Build history of the part. All positions in model axes, mm. A direction names the side the tool comes from. Round coordinates to 2 decimals unless told otherwise and drop trailing zeros. Write each loop counter-clockwise with the first axis right and the second up, starting at its lowest first coordinate (ties: lowest second). Pieces come first, ordered by that corner, then holes. Notation, with made-up numbers: M 24.5,55 L 79.5,55 A34 ccw 79.5,85 Z; hole C -10,33.5 d8. An arc over 180 degrees is marked long. Write item = value, one per line.
from build123d import *

# Parameters (mm, degrees)
ESQUISSE1_R             = 25
ESQUISSE1_R_2           = 1.7
BOSS_EXTRU_1_DEPTH      = 4
ESQUISSE11_R            = 1
ENL_V_MAT_EXTRU_1_DEPTH = 36.580893749
ESQUISSE13_W            = 4.903660669
ESQUISSE13_H            = 28.894120166
ENL_V_MAT_EXTRU_2_DEPTH = 36.580893749
ENL_V_MAT_EXTRU_3_DEPTH = 36.580893749


with BuildPart() as part:
    # Esquisse1 → Boss.-Extru.1 (new body)
    with BuildSketch(Plane.XY):
        Circle(ESQUISSE1_R)
        with Locations((-13.435028843, 13.435028843)):
            Circle(ESQUISSE1_R_2, mode=Mode.SUBTRACT)
        with Locations((13.435028843, 13.435028843)):
            Circle(ESQUISSE1_R_2, mode=Mode.SUBTRACT)
        with Locations((13.435028843, -13.435028843)):
            Circle(ESQUISSE1_R_2, mode=Mode.SUBTRACT)
        with Locations((-13.435028843, -13.435028843)):
            Circle(ESQUISSE1_R_2, mode=Mode.SUBTRACT)
    extrude(amount=BOSS_EXTRU_1_DEPTH)

    # Esquisse11 → Enlèv. mat.-Extru.1 (cut, through all)
    with BuildSketch(Plane(origin=(0, 0, 0), x_dir=(-1, 0, 0), z_dir=(0, 0, -1))):
        with Locations((0, 7.398882196)):
            Circle(ESQUISSE11_R)
        with Locations((5.827506735, 5.634287936)):
            Circle(ESQUISSE11_R)
        with Locations((5.827506735, -5.758693792)):
            Circle(ESQUISSE11_R)
        with Locations((0, -7.398882196)):
            Circle(ESQUISSE11_R)
        with Locations((-5.645080413, -5.758693792)):
            Circle(ESQUISSE11_R)
        with Locations((-5.645080413, 5.634287936)):
            Circle(ESQUISSE11_R)
    extrude(amount=-ENL_V_MAT_EXTRU_1_DEPTH, mode=Mode.SUBTRACT)

    # Esquisse13 → Enlèv. mat.-Extru.2 (cut, through all)
    with BuildSketch(Plane(origin=(0, 0, 0), x_dir=(-1, 0, 0), z_dir=(0, 0, -1))):
        with Locations((23.534998976, -1.01203124)):
            Rectangle(ESQUISSE13_W, ESQUISSE13_H)
    extrude(amount=-ENL_V_MAT_EXTRU_2_DEPTH, mode=Mode.SUBTRACT)

    # Esquisse10 → Enlèv. mat.-Extru.3 (cut, through all)
    with BuildSketch(Plane.XY.offset(4)):
        with BuildLine():
            Line((-5.758802096, -2.316766812), (-9.508802096, -5.566766812))
            ThreePointArc((-9.508802096, -5.566766812), (-10.566766812, -5.491197904), (-10.491197904, -4.433233188))
            Line((-10.491197904, -4.433233188), (-6.741197904, -1.183233188))
            ThreePointArc((-6.741197904, -1.183233188), (-5.683233188, -1.258802096), (-5.758802096, -2.316766812))
        make_face()
        with BuildLine():
            Line((-6.741197904, 1.183233188), (-10.491197904, 4.433233188))
            ThreePointArc((-10.491197904, 4.433233188), (-10.566766812, 5.491197904), (-9.508802096, 5.566766812))
            Line((-9.508802096, 5.566766812), (-5.758802096, 2.316766812))
            ThreePointArc((-5.758802096, 2.316766812), (-5.683233188, 1.258802096), (-6.741197904, 1.183233188))
        make_face()
        with BuildLine():
            Line((9.508802096, -5.566766812), (5.758802096, -2.316766812))
            ThreePointArc((5.758802096, -2.316766812), (5.683233188, -1.258802096), (6.741197904, -1.183233188))
            Line((6.741197904, -1.183233188), (10.491197904, -4.433233188))
            ThreePointArc((10.491197904, -4.433233188), (10.566766812, -5.491197904), (9.508802096, -5.566766812))
        make_face()
        with BuildLine():
            Line((10.491197904, 4.433233188), (6.741197904, 1.183233188))
            ThreePointArc((6.741197904, 1.183233188), (5.683233188, 1.258802096), (5.758802096, 2.316766812))
            Line((5.758802096, 2.316766812), (9.508802096, 5.566766812))
            ThreePointArc((9.508802096, 5.566766812), (10.566766812, 5.491197904), (10.491197904, 4.433233188))
        make_face()
    extrude(amount=-ENL_V_MAT_EXTRU_3_DEPTH, mode=Mode.SUBTRACT)


solid = part.part
1. Band-saw the part on C-C (y = 1.75). List the corners of the cut face in (x, z).
Responses:
outline = M -21.08,0 L -7.4,0 L -7.4,4 L -21.08,4 Z; M -5.5,0 L 5.5,0 L 5.5,4 L -5.5,4 Z; M 7.4,0 L 24.94,0 L 24.94,4 L 7.4,4 Z
2. Mould opens along Y. For faces 3 (the face through (-21.083, 0, 2)), 4 (the face through (8.64, 2.83, 2.03)), 5 (the face through (24.984, -0.901, 1.972)) say: pulls with the +Y half, pulls with the -Y half, needs draft (parallel to the pull), parting line crosses it, or undercut.
Responses:
face_3 = needs draft
face_4 = undercut
face_5 = parting line crosses it
3. Band-saw the part on A-A (x = 0). List the corners of the cut face in (y, z), plus the area to 3 significant figures.
Responses:
outline = M -25,0 L -8.4,0 L -8.4,4 L -25,4 Z; M -6.4,0 L 6.4,0 L 6.4,4 L -6.4,4 Z; M 8.4,0 L 25,0 L 25,4 L 8.4,4 Z
area = 184 mm²
4. Tool access for faces 1 (the face through (7.61, 3.92, 2.03)), 2 (the face through (2, 0, 0)): list every direction of +Z, -Z, +X, -X, +Y, -Y with a clear straight run to the whole face (end or side of a thin tool).
Responses:
face_1 = +Z, -Z
face_2 = -Z, +X, -X, +Y, -Y
5. Probe probe 1 along Y at (x, z) = (0, 2.3); probe 2 along Y at (x, z) = (9.5, 0.55); probe 3 along X at (y, z) = (13, 2.95). List the from-to ranges inside material, lowest first.
Responses:
probe_1 = -25 to -8.4, -6.4 to 6.4, 8.4 to 25
probe_2 = -23.12 to -5.56, -3.57 to 3.57, 5.56 to 23.12
probe_3 = -21.08 to -15.08, -11.79 to 11.79, 15.08 to 21.35
6. Band-saw the part on D-D (x = 20.5). List the corners of the cut face in (y, z).
Responses:
outline = M -14.31,0 L 14.31,0 L 14.31,4 L -14.31,4 Z
7. Flat gauge pins, fed straight in: pin 1 (2.5 mm diameter, centred on x = -13.44, y = -13.44, fed in from +Z); pin 2 (2 mm diameter, centred on x = 0, z = 1, fed in from -Y); pin 3 (1 mm diameter, centred on x = -15, z = 2.5, fed in from +Y). Where does each tip first touch, or does it go through?
Responses:
pin_1 = through
pin_2 = -25
pin_3 = 20.37
8. Band-saw the part on B-B (z = 0.95). Count the separate pieces of the cut face and the enclosed holes in it, plus the area to 3 significant figures.
Responses:
separate_pieces = 1
enclosed_holes = 14
area = 1,800 mm²
